Can you work these out from the model? Positions are in its coordinate system, mm. Face numbers are marked on the shaded views. A direction names the side the tool comes from. Give positions to 0.01 mm unless a question says otherwise; leave off trailing zeros. Loops run counter-clockwise (first coordinate to the right, second up) from the corner with the lowest first, then second, coordinate; pieces in that order, holes last. Notation, with made-up numbers: (44.25, 9.25) - (54.25, 9.25) arc R25 cw to (54.25, 42.25) - close; hole circle Ø7 at (60, -6). An arc over 180 degrees is marked (long way). Answer as a JSON object with one key per item and string values. Group by question number.
Item 1: Suppose I cut it at A-A on z = -7. Write out the boundary of the cut face in (x, y), and give its area (3 significant figures).
Item 2: Suppose I cut it at D-D on x = -26. Write out the boundary of the cut face in (y, z).
Item 3: Which directions (+Z, -Z, +X, -X, +Y, -Y) give clear straight access to the entire face, cutting with the end or side of a thin tool? Please do the marked faces 5, 6, 7 and 8.
Item 4: Suppose I cut it at B-B on x = 0. Write out the boundary of the cut face in (y, z), and give its area (3 significant figures).
Item 5: Please list where these lines run through material, in increasing order: L1, parallel to X at y = 0, z = -25.8; L2, parallel to X at y = -5, z = -7.25; L3, parallel to Y at x = 0, z = -25.9.
Item 6: Thinking about a two-plate mould opening in Z: for the marked faces 1, 2, 3 and 4, which applies, pulls with the +Z half, pulls with the -Z half, needs draft (parallel to the pull), parting line crosses it, or undercut?
Item 7: Will these pins go through, and if not, where does the flat tip stop? pin 1 (3.5 mm diameter, centred on y = 1, z = -17.5, fed in from +X); pin 2 (1 mm diameter, centred on y = 5.5, z = -20.5, fed in from -X); pin 3 (4 mm diameter, centred on x = 15.5, z = -20, fed in from -Y).
Item 8: Suppose I cut it at C-C on y = 0. Write out the boundary of the cut face in (x, z), and give its area (3 significant figures).
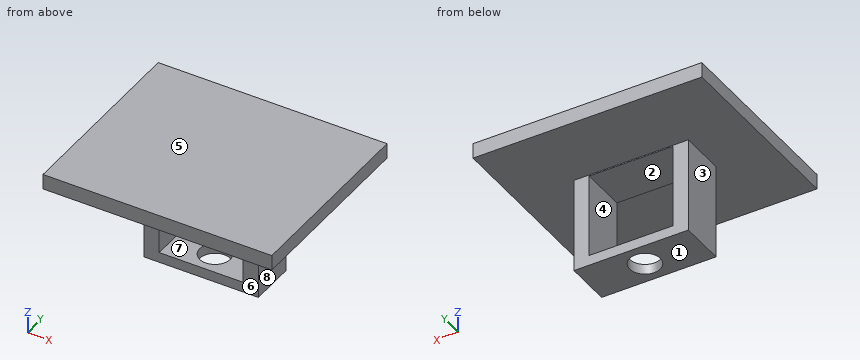
from build123d import *

# Parameters (mm, degrees)
F0_W          = 60
F0_H          = 4
F1_DEPTH      = 25
F1_DEPTH_BACK = 25
F2_W          = 30
F2_H          = 12
F3_DEPTH      = 25
F4_W          = 22
F4_H          = 22
F5_DEPTH      = 25
F6_R          = 4
F7_DEPTH      = 10


with BuildPart() as f1:
    # F0 (on Front) → F1 (new body, two sides)
    with BuildSketch(Plane.XZ) as f1_sk:
        Rectangle(F0_W, F0_H)
    extrude(amount=F1_DEPTH)
    extrude(f1_sk.sketch, amount=-F1_DEPTH_BACK)

    # F2 (on face) → F3 (join)
    with BuildSketch(Plane(origin=(0, 0, -2), x_dir=(1, 0, 0), z_dir=(0, 0, -1))):
        Rectangle(F2_W, F2_H)
    extrude(amount=F3_DEPTH)

    # F4 (on face) → F5 (cut)
    with BuildSketch(Plane(origin=(0, 6, 0), x_dir=(-1, 0, 0), z_dir=(0, 1, 0))):
        with Locations((0, -13.310707)):
            Rectangle(F4_W, F4_H)
    extrude(amount=-F5_DEPTH, mode=Mode.SUBTRACT)

    # F6 (on face) → F7 (cut)
    with BuildSketch(Plane(origin=(0, 0, -27), x_dir=(1, 0, 0), z_dir=(0, 0, -1))):
        Circle(F6_R)
    extrude(amount=-F7_DEPTH, mode=Mode.SUBTRACT)


solid = f1.part
Worked out:
{
 "1": {"outline": "(-15, -6) - (-11, -6) - (-11, 6) - (-15, 6) - close; (11, -6) - (15, -6) - (15, 6) - (11, 6) - close", "area": "96.0 mm2"},
 "2": {"outline": "(-25, -2) - (25, -2) - (25, 2) - (-25, 2) - close"},
 "3": {"face 5": "+Z, +X, -X, +Y, -Y", "face 6": "-Z, +X, -X, -Y", "face 7": "+Y, -Y", "face 8": "-Z, +X, +Y, -Y"},
 "4": {"outline": "(-25, -2) - (-6, -2) - (-6, -2.31) - (6, -2.31) - (6, -2) - (25, -2) - (25, 2) - (-25, 2) - close; (-6, -27) - (-4, -27) - (-4, -24.31) - (-6, -24.31) - close; (4, -27) - (6, -27) - (6, -24.31) - (4, -24.31) - close", "area": "214 mm2"},
 "5": {"L1": "x = -15 to -4, 4 to 15", "L2": "x = -15 to -11, 11 to 15", "L3": "y = -6 to -4, 4 to 6"},
 "6": {"face 1": "pulls with the -Z half", "face 2": "undercut", "face 3": "needs draft", "face 4": "undercut"},
 "7": {"pin 1": "stops at x = 15", "pin 2": "stops at x = -15", "pin 3": "stops at y = -6"},
 "8": {"outline": "(-30, -2) - (-15, -2) - (-15, -27) - (-4, -27) - (-4, -24.31) - (-11, -24.31) - (-11, -2.31) - (11, -2.31) - (11, -24.31) - (4, -24.31) - (4, -27) - (15, -27) - (15, -2) - (30, -2) - (30, 2) - (-30, 2) - close", "area": "484 mm2"}
}
